```python
from build123d import *

# Parameters (mm, degrees)
F1_DEPTH = 1000
F2_R     = 5


with BuildPart() as f1:
    # F0 (on Right) → F1 (new body)
    with BuildSketch(Plane.YZ):
        with BuildLine():
            Line((-20, -12.5), (20, -12.5))
            ThreePointArc((20, -12.5), (23.5355339059, -11.0355339059), (25, -7.5))
            Line((25, -7.5), (25, 7.5))
            ThreePointArc((25, 7.5), (23.5355339059, 11.0355339059), (20, 12.5))
            Line((20, 12.5), (-20, 12.5))
            ThreePointArc((-20, 12.5), (-23.5355339059, 11.0355339059), (-25, 7.5))
            Line((-25, 7.5), (-25, -7.5))
            ThreePointArc((-25, -7.5), (-23.5355339059, -11.0355339059), (-20, -12.5))
        make_face()
    extrude(amount=F1_DEPTH)

    # F2
    f2_edges = [f1.edges().sort_by_distance(p)[0] for p in [
        (1000, -25, 0),
        (0, 25, 0),
    ]]
    fillet(f2_edges, radius=F2_R)


solid = f1.part
```
Can you work these out from the model? Positions are in its coordinate system, mm. Coordinates: 2 decimals unless noted, no trailing zeros. Order: outer loops, then holes, each group sorted by start corner. A loop starts at its lowest first (then second) coordinate and runs counter-clockwise, first axis right, second up.
1. I need wall thicknesses on line 1 (Y direction, x = 135, z = -8.5); line 2 (Z direction, x = 90, y = -21); line 3 (X direction, y = -23, z = 6). Which ranges of each line are inside material? Lowest first, please.
2. I'm going to push a flat-ended pin straight in: pin 1 (1 mm diameter, centred on y = -14, z = -8.5, fed in from +X). Where does the tip first touch, or does it pass through?
3. If we section it at A-A (x = 193): Please give me the cut outline in (y, z).
Entries:
1. line 1: y = -24.9 to 24.9
1. line 2: z = -12.4 to 12.4
1. line 3: x = 1 to 999
2. pin 1: stops at x = 999.97
3. outline: (-25, -7.5) arc R5 ccw to (-20, -12.5) - (20, -12.5) arc R5 ccw to (25, -7.5) - (25, 7.5) arc R5 ccw to (20, 12.5) - (-20, 12.5) arc R5 ccw to (-25, 7.5) - close
